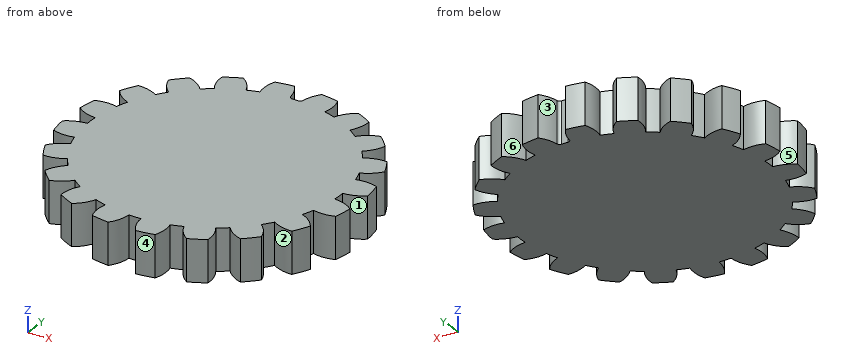
from build123d import *

# Parameters (mm, degrees)
SKETCH1_R           = 17.5
BOSS_EXTRUDE1_DEPTH = 2.5
CUT_EXTRUDE1_DEPTH  = 25.874685928
FILLET2_R           = 0.375
CIRPATTERN1_COUNT   = 20


with BuildPart() as part:
    # Sketch1 → Boss-Extrude1 (new, symmetric)
    with BuildSketch(Plane.XY):
        Circle(SKETCH1_R)
    extrude(amount=BOSS_EXTRUDE1_DEPTH, both=True)

    # Sketch3 → Cut-Extrude1 (cut, symmetric)
    with BuildSketch(Plane.XY):
        with BuildLine():
            ThreePointArc((-2.639096151, 18.310793852), (-1.2854332, 16.875635392), (-0.731537344, 14.982151151))
            ThreePointArc((-0.731537344, 14.982151151), (0, 15), (0.731537344, 14.982151151))
            ThreePointArc((0.731537344, 14.982151151), (1.2854332, 16.875635392), (2.639096151, 18.310793852))
            ThreePointArc((2.639096151, 18.310793852), (0, 18.5), (-2.639096151, 18.310793852))
        make_face()
    cut_extrude1 = extrude(amount=CUT_EXTRUDE1_DEPTH, both=True, mode=Mode.SUBTRACT)

    # Fillet2
    fillet2_edges = [part.edges().sort_by_distance(p)[0] for p in [
        (-0.731537344, 14.982151151, 0),
        (0.731537344, 14.982151151, 0),
    ]]
    fillet(fillet2_edges, radius=FILLET2_R)

    # CirPattern1: Cut-Extrude1 ×20 about axis
    cirpattern1_axis = Axis((0, 0, 0), (0, 0, 1))
    for i in range(1, CIRPATTERN1_COUNT):
        add(cut_extrude1.rotate(cirpattern1_axis, i * 360 / CIRPATTERN1_COUNT), mode=Mode.SUBTRACT)


solid = part.part
Can you work these out from the model? Positions are in its coordinate system, mm. Face numbers are marked on the shaded views. A direction names the side the tool comes from. Give positions to 0.01 mm unless a question says otherwise; leave off trailing zeros. Loops run counter-clockwise (first coordinate to the right, second up) from the corner with the lowest first, then second, coordinate; pieces in that order, holes last. Notation, with made-up numbers: (-28, 23.25) - (19, 23.25) arc R11 ccw to (19, 43.25) - close; hole circle Ø3 at (-12, 21). An arc over 180 degrees is marked (long way). Answer as a JSON object with one key per item and string values.
Q1. If I drill on L1, parallel to Y at x = -12, z = 0.85; L2, parallel to Y at x = 14.5, z = 1.15, over which ranges is the centre line in solid material (lowest first)?
Geometry says:
{"L1": "-12.74 to -9.67, -9 to 9, 9.67 to 12.74", "L2": "-8.89 to -5.54, -3.94 to 3.94, 5.54 to 8.89"}
Q2. If we mould it in two halves opening along X, with no side actions, what happens to the marked faces 4, 5 and 6? For each: pulls with the +X half, pulls with the -X half, needs draft (parallel to the pull), parting line crosses it, or undercut.
Geometry says:
{"face 4": "pulls with the +X half", "face 5": "pulls with the -X half", "face 6": "undercut"}
Q3. Imagine slicing it at A-A on y = -10.5. Write out the boundary of the cut face in (x, z), plus the area to 3 significant figures.
Geometry says:
{"outline": "(-12.66, -2.5) - (12.66, -2.5) - (12.66, 2.5) - (-12.66, 2.5) - close", "area": "127 mm²"}
Q4. Which directions (+Z, -Z, +X, -X, +Y, -Y) give clear straight access to the entire face, cutting with the end or side of a thin tool? Please do the marked faces 1, 2 and 3.
Geometry says:
{"face 1": "+Z, -Z, +X", "face 2": "+Z, -Z", "face 3": "+Z, -Z, +Y"}
Q5. Imagine slicing it at B-B on x = -6. Write out the boundary of the cut face in (y, z), plus the area to 3 significant figures.
Geometry says:
{"outline": "(-15.19, -2.5) - (15.19, -2.5) - (15.19, 2.5) - (-15.19, 2.5) - close", "area": "152 mm²"}
Q6. Will this pin go through, and if not, where does the flat tip stop? P1, Ø3, axis at x = -9, z = 1.5, coming from the +Y side.
Geometry says:
{"P1": "y = 15.81"}
